Part model, mm, in its own coordinate system. Round coordinates to 2 decimals unless told otherwise and drop trailing zeros. Order: outer loops, then holes, each group sorted by start corner. A loop starts at its lowest first (then second) coordinate and runs counter-clockwise, first axis right, second up. Notation, with made-up numbers: (48, -9.75) -> (100, -9.75) arc R34 ccw to (100, 23.25) -> close; hole circle Ø2 at (63.5, -25). An arc over 180 degrees is marked (long way). Use CSV: the item, a comma, the result in double quotes.
```python
from build123d import *

# Parameters (mm, degrees)
CROQUIS1_R              = 50
CROQUIS1_R_2            = 5
SALIENTE_EXTRUIR1_DEPTH = 10


with BuildPart() as part:
    # Croquis1 → Saliente-Extruir1 (new body)
    with BuildSketch(Plane.XY):
        Circle(CROQUIS1_R)
        with Locations((-37.977099237, 0)):
            Circle(CROQUIS1_R_2, mode=Mode.SUBTRACT)
        with Locations((-34.693806502, 15.446677857)):
            Circle(CROQUIS1_R_2, mode=Mode.SUBTRACT)
        with Locations((-25.41163944, 28.222484784)):
            Circle(CROQUIS1_R_2, mode=Mode.SUBTRACT)
        with Locations((-11.735569061, 36.118367699)):
            Circle(CROQUIS1_R_2, mode=Mode.SUBTRACT)
        with Locations((3.969687823, 37.769056713)):
            Circle(CROQUIS1_R_2, mode=Mode.SUBTRACT)
        with Locations((18.988549618, 32.889132701)):
            Circle(CROQUIS1_R_2, mode=Mode.SUBTRACT)
        with Locations((30.72411868, 22.322378856)):
            Circle(CROQUIS1_R_2, mode=Mode.SUBTRACT)
        with Locations((37.147208501, 7.895882915)):
            Circle(CROQUIS1_R_2, mode=Mode.SUBTRACT)
        with Locations((37.147208501, -7.895882915)):
            Circle(CROQUIS1_R_2, mode=Mode.SUBTRACT)
        with Locations((30.72411868, -22.322378856)):
            Circle(CROQUIS1_R_2, mode=Mode.SUBTRACT)
        with Locations((18.988549618, -32.889132701)):
            Circle(CROQUIS1_R_2, mode=Mode.SUBTRACT)
        with Locations((3.969687823, -37.769056713)):
            Circle(CROQUIS1_R_2, mode=Mode.SUBTRACT)
        with Locations((-11.735569061, -36.118367699)):
            Circle(CROQUIS1_R_2, mode=Mode.SUBTRACT)
        with Locations((-25.41163944, -28.222484784)):
            Circle(CROQUIS1_R_2, mode=Mode.SUBTRACT)
        with Locations((-34.693806502, -15.446677857)):
            Circle(CROQUIS1_R_2, mode=Mode.SUBTRACT)
    extrude(amount=SALIENTE_EXTRUIR1_DEPTH)


solid = part.part
```
(1) Drop flat-ended pins along their axis: P1, Ø1, axis at y = 32, z = 1.5, coming from the -X side; P2, Ø4, axis at y = 25, z = 6, coming from the -X side; P3, Ø1.5, axis at y = 10, z = 4, coming from the -X side. Give the stop position or say it passes through.
Reply:
P1,"x = -38.83"
P2,"x = -44.4"
P3,"x = -49.14"
(2) Cut at D-D, the plane x = 10.5. Give the cut face in (y, z), then the cut area to 3 significant figures.
Reply:
outline,"(-48.89, 0) -> (48.89, 0) -> (48.89, 10) -> (-48.89, 10) -> close"
area,"978 mm2"
(3) Cut at B-B, the plane x = -15.5. Give the cut face in (y, z), then the cut area to 3 significant figures.
Reply:
outline,"(-47.54, 0) -> (-39.41, 0) -> (-39.41, 10) -> (-47.54, 10) -> close; (-32.83, 0) -> (32.83, 0) -> (32.83, 10) -> (-32.83, 10) -> close; (39.41, 0) -> (47.54, 0) -> (47.54, 10) -> (39.41, 10) -> close"
area,"819 mm2"
(4) Probe probe 1 along X at (y, z) = (-31, 9); probe 2 along X at (y, z) = (-26, 1.25); probe 3 along Y at (x, z) = (17.5, 5.75). List the from-to ranges inside material, lowest first. Write a range as [from, to].
Reply:
probe 1,"[-39.23, -29.57], [-21.25, 14.36], [23.62, 39.23]"
probe 2,"[-42.71, -29.89], [-20.93, 27.34], [34.11, 42.71]"
probe 3,"[-46.84, -37.66], [-28.12, 28.12], [37.66, 46.84]"
(5) Cut at C-C, the plane z = 3.5. State how many separate pieces and enclosed holes the cut face has, then the cut area to 3 significant figures.
Reply:
separate pieces,"1"
enclosed holes,"15"
area,"6,680 mm2"
(6) Cut at A-A, the plane y = 0. Give the cut face in (x, z), then the cut area to 3 significant figures.
Reply:
outline,"(-50, 0) -> (-42.98, 0) -> (-42.98, 10) -> (-50, 10) -> close; (-32.98, 0) -> (50, 0) -> (50, 10) -> (-32.98, 10) -> close"
area,"900 mm2"
(7) Pull direction X, two halves, no side cores. Call faces 1 (the face through (47.69, 15.02, 4.93)), 2 (the face through (-1, 1, 10)), 3 (the face through (8.59, -39.68, 4.93)): released by +X, released by -X, zero draft, split by the parting line, or undercut.
Reply:
face 1,"split by the parting line"
face 2,"zero draft"
face 3,"undercut"
